Check sheet for the modelled part. Datum: model origin and axes. Units: mm. Round coordinates to 2 decimals unless told otherwise and drop trailing zeros. Write each loop counter-clockwise with the first axis right and the second up, starting at its lowest first coordinate (ties: lowest second). Pieces come first, ordered by that corner, then holes. Notation, with made-up numbers: M 7.5,12.5 L 30.5,12.5 A16 cw 30.5,24.5 Z; hole C 41,-2 d3. An arc over 180 degrees is marked long. Put each result on its own line as item: value.
Autodesk Inventor part; units mm, degrees
ref_plane "YZ Plane" through (0, 0, 0) normal (1, 0, 0) x (0, 1, 0)
ref_plane "XZ Plane" through (0, 0, 0) normal (0, 1, 0) x (-1, 0, 0)
ref_plane "XY Plane" through (0, 0, 0) normal (0, 0, 1) x (1, 0, 0)
sketch "スケッチ1" plane through (0, 0, 0) normal (0, 0, 1) x (1, 0, 0)
  line L0 (50, -27.5) -> (-50, -27.5)
  line L1 (-50, -27.5) -> (-50, 27.5)
  line L2 (-50, 27.5) -> (50, 27.5)
  line L3 (50, 27.5) -> (50, -27.5)
  line L4 (50, -27.5) -> (-50, 27.5) construction
  line L5 (-50, -27.5) -> (50, 27.5) construction
  circle A0 centre (0, 0) radius 25
  line L6 (-50, 0) -> (50, 0)
  circle A1 centre (25, 0) radius 9
  circle A2 centre (-25, 0) radius 12.5
  circle A3 centre (-25, 0) radius 17.5
  circle A4 centre (-25, 17.5) radius 2.05
  circle A5 centre (-42.5, 0) radius 2.05
  circle A6 centre (-25, -17.5) radius 2.05
  circle A7 centre (-7.5, 0) radius 2.05
  dimension "d5" = 35
  dimension "d0" = 100
  dimension "d1" = 55
  dimension "d2" = 50
  dimension "d3" = 18
  dimension "d4" = 25
  dimension "d6" = 4.1
  dimension "d9" = 360
  dimension "d11" = 25
extrude "押し出し1" add sketch "スケッチ1" along normal blind 3 contours L0 L1 L6 A5 A3 A6 A0 A1 L3 | L6 A1 A0 A3 A4 A5 L1 L2 L3 | A5 A3 L6 | L6 A3 A5 | A1 L6 A7 A3 A0 | A0 A3 A7 L6 A1 | A3 A5 L6 | L6 A5 A3 | A3 A4 A0 A2 L6 A5 | A5 L6 A2 A0 A3 A6 | A3 A7 L6 A2 A0 | A0 A2 L6 A7 A3 | A4 A3 | A3 A4 | A6 A3 | A3 A6 | A7 A3 L6 | L6 A3 A7 | A2 L6 A0 | A0 L6 A2 | A3 L6 A7 | A2 L6 A0 | A0 L6 A2 | A7 L6 A3
sketch "スケッチ2" plane through (0, 0, 3) normal (0, 0, 1) x (1, 0, 0)
  line L0 (50, 27.5) -> (-50, 27.5)
  line L1 (-50, 27.5) -> (-50, -27.5)
  line L2 (-50, -27.5) -> (50, -27.5)
  line L3 (50, -27.5) -> (50, 27.5)
  circle A0 centre (25, 0) radius 9
  line L4 (-45, 22.5) -> (45, 22.5)
  line L5 (45, 22.5) -> (45, -22.5)
  line L6 (45, -22.5) -> (-45, -22.5)
  line L7 (-45, -22.5) -> (-45, 22.5)
  point P0 (0, 0)
  dimension "d14" = 5
hole "穴1" at (-45, 22.5, 3) at (-45, -22.5, 3) at (45, -22.5, 3) at (45, 22.5, 3) direction (0, 0, -1) diameter 3.2 end through all
fillet "フィレット1" radius 2 4 edges at (-50, 27.5, 1.5) (50, 27.5, 1.5) (50, -27.5, 1.5) (-50, -27.5, 1.5)
sketch "スケッチ3" plane through (0, 0, 3) normal (0, 0, 1) x (1, 0, 0)
  arc A0 (-50, -25.5) -> (-48, -27.5) centre (-48, -25.5) ccw
  line L0 (-48, -27.5) -> (48, -27.5)
  arc A1 (48, -27.5) -> (50, -25.5) centre (48, -25.5) ccw
  line L1 (50, -25.5) -> (50, 25.5)
  arc A2 (50, 25.5) -> (48, 27.5) centre (48, 25.5) ccw
  line L2 (48, 27.5) -> (-48, 27.5)
  arc A3 (-48, 27.5) -> (-50, 25.5) centre (-48, 25.5) ccw
  line L3 (-50, 25.5) -> (-50, -25.5)
  circle A4 centre (45, 22.5) radius 1.6
  circle A5 centre (45, -22.5) radius 1.6
  circle A6 centre (-45, -22.5) radius 1.6
  circle A7 centre (-45, 22.5) radius 1.6
  circle A8 centre (25, 0) radius 9
  point P0 (0, 0)
equation "\"d11\" = -0.5 * d2 + 0.5 * d0"
properties part number "xx_plate_nomotor"
1. Release check for a two-part mould opening along X. For faces 1 (the cylindrical face through (-49.4, 26.93, 1.52)), 2 (the cylindrical face through (49.43, 26.9, 1.52)), 3 (the cylindrical face through (46.42, 21.76, 1.48)) record: +X half, -X half, draft (parallel to the pull), parting line (faces both ways), or undercut.
Computed values:
face 1: -X half
face 2: +X half
face 3: undercut
2. Cross-section at C-C (x = -45). Enter the section's corners in (y, z).
Computed values:
outline: M -27.5,0 L -24.1,0 L -24.1,3 L -27.5,3 Z; M -20.9,0 L 20.9,0 L 20.9,3 L -20.9,3 Z; M 24.1,0 L 27.5,0 L 27.5,3 L 24.1,3 Z
3. Scan lines: probe 1 along X at (y, z) = (22.5, 2.35); probe 2 along Y at (x, z) = (45, 1.3); probe 3 along X at (y, z) = (0, 1.1). Record each from-to range of solid material in increasing order.
Computed values:
probe 1: x = -50 to -46.6, -43.4 to 43.4, 46.6 to 50
probe 2: y = -27.5 to -24.1, -20.9 to 20.9, 24.1 to 27.5
probe 3: x = -50 to 16, 34 to 50
4. Depth check by flat-ended pin: pin 1 Ø14.5 at (x, y) = (25, 0) entering from -Z. Enter the tip coordinate at first touch or a pass-through.
Computed values:
pin 1: passes through
5. Cross-section at D-D (x = 25). Enter the section's corners in (y, z).
Computed values:
outline: M -27.5,0 L -9,0 L -9,3 L -27.5,3 Z; M 9,0 L 27.5,0 L 27.5,3 L 9,3 Z
6. Cross-section at A-A (y = 0). Enter the section's corners in (x, z), then the cut area to 3 significant figures.
Computed values:
outline: M -50,0 L 16,0 L 16,3 L -50,3 Z; M 34,0 L 50,0 L 50,3 L 34,3 Z
area: 246 mm2
7. Cross-section at B-B (z = 1). Enter the section's corners in (x, y).
Computed values:
outline: M -50,-25.5 A2 ccw -48,-27.5 L 48,-27.5 A2 ccw 50,-25.5 L 50,25.5 A2 ccw 48,27.5 L -48,27.5 A2 ccw -50,25.5 Z; hole C -45,-22.5 d3.2; hole C -45,22.5 d3.2; hole C 25,0 d18; hole C 45,-22.5 d3.2; hole C 45,22.5 d3.2
